```python
from build123d import *

# Parameters (mm, degrees)
F0_R     = 0.9525
F0_R_2   = 2.5527
F0_R_3   = 3.175
F1_DEPTH = 3.175
F2_R     = 6.35
F2_R_2   = 2.5527
F3_DEPTH = 3.175


with BuildPart() as f1:
    # F0 (on Front) → F1 (new body)
    with BuildSketch(Plane.XZ):
        with BuildLine():
            Line((-2.766543, 10.495013), (-22.020772, 6.197504))
            ThreePointArc((-22.020772, 6.197504), (-26.9875, 0), (-22.020772, -6.197504))
            Line((-22.020772, -6.197504), (-2.766543, -10.495013))
            ThreePointArc((-2.766543, -10.495013), (0, -10.800004), (2.766543, -10.495013))
            Line((2.766543, -10.495013), (22.020772, -6.197504))
            ThreePointArc((22.020772, -6.197504), (26.9875, 0), (22.020772, 6.197504))
            Line((22.020772, 6.197504), (2.766543, 10.495013))
            ThreePointArc((2.766543, 10.495013), (0, 10.800004), (-2.766543, 10.495013))
        make_face()
        with Locations((5.26243, -5.26243)):
            Circle(F0_R, mode=Mode.SUBTRACT)
        with Locations((-20.6375, 0)):
            Circle(F0_R_2, mode=Mode.SUBTRACT)
        with Locations((-5.26243, 5.26243)):
            Circle(F0_R, mode=Mode.SUBTRACT)
        Circle(F0_R_3, mode=Mode.SUBTRACT)
        with Locations((20.6375, 0)):
            Circle(F0_R_2, mode=Mode.SUBTRACT)
    extrude(amount=F1_DEPTH)

    # F2 (on face) → F3 (join)
    with BuildSketch(Plane.XZ.offset(3.175)):
        with Locations((20.6375, 0)):
            Circle(F2_R)
        with Locations((20.6375, 0)):
            Circle(F2_R_2, mode=Mode.SUBTRACT)
        with Locations((-20.6375, 0)):
            Circle(F2_R)
        with Locations((-20.6375, 0)):
            Circle(F2_R_2, mode=Mode.SUBTRACT)
    extrude(amount=F3_DEPTH)


solid = f1.part
```
Verification items for the finished model (mm, model axes). Give positions to 0.01 mm unless a question says otherwise; leave off trailing zeros. Order: outer loops, then holes, each group sorted by start corner. A loop starts at its lowest first (then second) coordinate and runs counter-clockwise, first axis right, second up. Notation, with made-up numbers: (70, -1) -> (112, -1) arc R22 cw to (112, 22) -> close; hole circle Ø9 at (59, -30.75). An arc over 180 degrees is marked (long way). One line per item, written item: value.
(1) Sectioned sample at B-B on x = 0. Record the cut outline in (y, z) (3 decimals).
Final values:
outline: (-3.175, -10.8) -> (0, -10.8) -> (0, -3.175) -> (-3.175, -3.175) -> close; (-3.175, 3.175) -> (0, 3.175) -> (0, 10.8) -> (-3.175, 10.8) -> close
(2) Draft check along Z on faces 1 (the face through (12.528, -1.565, 8.316)), 2 (the face through (22.996, -3.131, -0.978)), 3 (the face through (-12.528, -1.565, -8.316)), 4 (the face through (6.14, -1.57, -5.63)). Enter one of: pulls with the +Z half, pulls with the -Z half, needs draft (parallel to the pull), parting line crosses it, or undercut.
Final values:
face 1: pulls with the +Z half
face 2: undercut
face 3: pulls with the -Z half
face 4: undercut
(3) Sectioned sample at C-C on y = -5.75. Record the cut outline in (x, z).
Final values:
outline: circle Ø12.7 at (-20.64, 0); circle Ø12.7 at (20.64, 0); hole circle Ø5.11 at (-20.64, 0); hole circle Ø5.11 at (20.64, 0)
(4) Sectioned sample at A-A on z = 0. Count the separate pieces of the cut face and the enclosed holes in it, then the cut area to 3 significant figures.
Final values:
separate pieces: 4
enclosed holes: 0
area: 167 mm^2
(5) Scan lines: line 1 along X through (y, z) = (-5.75, -2.25); line 2 along X through (y, z) = (-0.25, 2); line 3 along Y through (x, z) = (2, 3.75) (3 decimals). Record each from-to range of solid material in increasing order. Write a range as [from, to].
Final values:
line 1: [-26.58, -21.84], [-19.43, -14.7], [14.7, 19.43], [21.84, 26.58]
line 2: [-26.66, -22.22], [-19.05, -2.47], [2.47, 19.05], [22.22, 26.66]
line 3: [-3.175, 0]
(6) Gauge pin test, flat ends, axial feed: pin 1 (1.7 mm diameter, centred on x = 5.26, z = -5.26, fed in from +Y); pin 2 (11 mm diameter, centred on x = 2.5, z = 1.5, fed in from -Y) (3 decimals); pin 3 (1 mm diameter, centred on y = -5, z = -4.5, fed in from +X); pin 4 (1.5 mm diameter, centred on y = -4.5, z = 5.5, fed in from +X). Record the tip position at first contact, or that the pin passes through.
Final values:
pin 1: through
pin 2: y = -3.175
pin 3: x = 25.57
pin 4: x = 24.85
